For this review, use the dimensioned drawing (mm, ordinates from the lowest corner) and the shaded views. A direction names the side the tool comes from. Give positions to 0.01 mm unless a question says otherwise; leave off trailing zeros. Order: outer loops, then holes, each group sorted by start corner. A loop starts at its lowest first (then second) coordinate and runs counter-clockwise, first axis right, second up. Notation, with made-up numbers: (-30, 77) -> (29, 77) arc R11 ccw to (29, 86) -> close; hole circle Ø8 at (-24.5, -21.75). An arc over 180 degrees is marked (long way). Return JSON: item names as keys, results as strings.
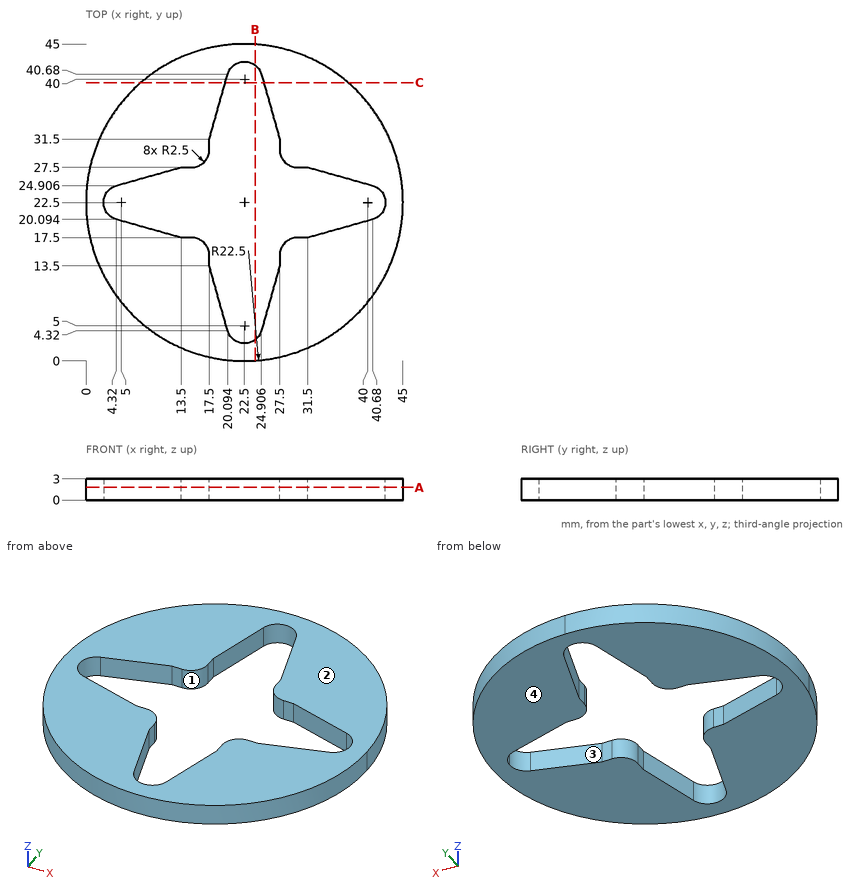
Item 1: Mouldability with a two-part tool opening along X and no side actions: class the marked faces 1 and 2 as released by +X, released by -X, zero draft, split by the parting line, or undercut.
Result set:
{"face 1": "undercut", "face 2": "zero draft"}
Item 2: Machinability: for the marked faces 3 and 4, which of the approach directions +Z, -Z, +X, -X, +Y, -Y give a long, thin tool a straight path to every point of the face, cutting with its end or side? Answer none if there is none.
Result set:
{"face 3": "+Z, -Z", "face 4": "-Z, +X, -X, +Y, -Y"}
Item 3: Wall thickness on L1, parallel to X at y = 35, z = 0.5; L2, parallel to X at y = 3, z = 2.6 (1 decimal); L3, parallel to Y at x = 30.5, z = 1.4: over which ranges is each line inside the solid? List them lowest first. Write a range as [from, to].
Result set:
{"L1": "x = [3.79, 18.49], [26.51, 41.21]", "L2": "x = [11.3, 21], [24, 33.7]", "L3": "y = [1.47, 17.5], [27.5, 43.53]"}
Item 4: Add section C-C (y = 39.5). Give the boundary of the cut face in (x, z).
Result set:
{"outline": "(7.76, 0) -> (19.76, 0) -> (19.76, 3) -> (7.76, 3) -> close; (25.24, 0) -> (37.24, 0) -> (37.24, 3) -> (25.24, 3) -> close"}
Item 5: Add section A-A (z = 1.8). Give the boundary of the cut face in (x, y) (1 decimal).
Result set:
{"outline": "circle Ø45 at (22.5, 22.5); hole (4.3, 20.1) -> (13.5, 17.5) -> (15, 17.5) arc R2.5 cw to (17.5, 15) -> (17.5, 13.5) -> (20.1, 4.3) arc R2.5 ccw to (24.9, 4.3) -> (27.5, 13.5) -> (27.5, 15) arc R2.5 cw to (30, 17.5) -> (31.5, 17.5) -> (40.7, 20.1) arc R2.5 ccw to (40.7, 24.9) -> (31.5, 27.5) -> (30, 27.5) arc R2.5 cw to (27.5, 30) -> (27.5, 31.5) -> (24.9, 40.7) arc R2.5 ccw to (20.1, 40.7) -> (17.5, 31.5) -> (17.5, 30) arc R2.5 cw to (15, 27.5) -> (13.5, 27.5) -> (4.3, 24.9) arc R2.5 ccw to start"}
Item 6: Add section B-B (x = 24). Give the boundary of the cut face in (y, z).
Result set:
{"outline": "(0.05, 0) -> (3, 0) -> (3, 3) -> (0.05, 3) -> close; (42, 0) -> (44.95, 0) -> (44.95, 3) -> (42, 3) -> close"}
Item 7: For pin 1 (1.6 mm diameter, centred on x = 14, z = 1, fed in from +Y); pin 2 (1.2 mm diameter, centred on y = 14.5, z = 1, fed in from -X); pin 3 (0.8 mm diameter, centred on x = 30.5, z = 1, fed in from -Y), all flat-tipped, find the tip position at first contact; note any pin that passes through.
Result set:
{"pin 1": "stops at y = 43.64", "pin 2": "stops at x = 1.25", "pin 3": "stops at y = 1.32"}
